The model under review builds one solid part; all positions refer to its coordinate system, in mm. A direction names the side the tool comes from. Coordinates: 2 decimals unless noted, no trailing zeros. Write each loop counter-clockwise with the first axis right and the second up, starting at its lowest first coordinate (ties: lowest second). Pieces come first, ordered by that corner, then holes. Notation, with made-up numbers: (60.5, 65.5) -> (66.5, 65.5) arc R32 cw to (66.5, 98.5) -> close; hole circle Ø2 at (46, -18.75). An arc over 180 degrees is marked (long way). Put each result on its own line as item: value. Start each with the question number.
Autodesk Inventor part; units mm, degrees
ref_plane "YZ Plane" through (0, 0, 0) normal (1, 0, 0) x (0, 1, 0)
ref_plane "XZ Plane" through (0, 0, 0) normal (0, 1, 0) x (-1, 0, 0)
ref_plane "XY Plane" through (0, 0, 0) normal (0, 0, 1) x (1, 0, 0)
sketch "Sketch1" plane through (0, 0, 0) normal (0, 0, 1) x (1, 0, 0)
  line L0 (0, 0) -> (-22, 0)
  line L1 (-22, 0) -> (-22, -15.6)
  line L2 (-22, -15.6) -> (-19, -15.6)
  line L3 (-19, -15.6) -> (-19, -5)
  line L4 (-19, -5) -> (-10, -5)
  line L5 (-10, -5) -> (-10, -2)
  line L6 (-10, -2) -> (0, -2)
  line L7 (0, -2) -> (0, 0)
  dimension "d0" = 2
  dimension "d1" = 10
  dimension "d2" = 3
  dimension "d3" = 9
  dimension "d4" = 3
  dimension "d5" = 10.6
extrude "Extrusion1" add sketch "Sketch1" along normal blind 10
chamfer "Chamfer1" distance 2 angle 45 1 edges at (-19, -5, 5)
sketch "Sketch2" plane through (-22, 0, 0) normal (0, 1, 0) x (1, 0, 0)
  line L0 (12, 0) -> (12, -10)
  line L1 (16.25, -5) -> (17.75, -5) construction
  line L2 (16.25, -6.75) -> (17.75, -6.75)
  line L3 (17.75, -3.25) -> (16.25, -3.25)
  arc A0 (16.25, -3.25) -> (16.25, -6.75) centre (16.25, -5) ccw
  arc A1 (17.75, -6.75) -> (17.75, -3.25) centre (17.75, -5) ccw
  point P0 (22, 0)
  point P1 (17, -5)
  dimension "d11" = 1.75
  dimension "d12" = 1.5
  dimension "d13" = 5
extrude "Extrusion2" cut sketch "Sketch2" against normal through all
chamfer "Chamfer2" distance 2 angle 45 1 edges at (-22, 0, 5)
chamfer "Chamfer3" distance 1 angle 45 8 edges at (-10, 0, 10) (-10, 0, 0) (0, 0, 5) (-21, -1, 10) (-22, -8.8, 10) (-21, -1, 0) (-22, -8.8, 0) (-22, -15.6, 5)
properties part number "_3DPrint"
1. Consider section A-A on z = 5. State the section outline as (x, y) points, then the cut area to 3 significant figures.
2. Consider section D-D on z = 2. State the section outline as (x, y) points, then the cut area to 3 significant figures.
3. Consider section C-C on x = -1.75. State the section outline as (y, z) points, then the cut area to 3 significant figures.
4. Insertion check: P1, Ø4, axis at y = -12, z = 8.5, coming from the +X side; P2, Ø0.9, axis at y = -4, z = 6.5, coming from the +X side. Each pin has a flat end and moves straight along its axis. Give the tip position at first contact, or say it passes through.
5. Tool access review of faces 5 (the cylindrical face through (-2.5, -1, 5)), 6 (the flat face through (-0.5, -0.5, 4.9)), 7 (the flat face through (-19, -11, 5)): name each direction out of +Z, -Z, +X, -X, +Y, -Y from which nothing blocks a thin tool from reaching the whole face with its end or side.
6. Wall thickness on line 1 (X direction, y = -4, z = 7); line 2 (X direction, y = -13, z = 4); line 3 (Y direction, x = -15.5, z = 2.25): over which ranges is each line inside the solid? List them lowest first. Write a range as from..to.
7. The part is to be moulded in two halves that separate along Z. For faces 1 (the flat face through (-16, -4, 0)), 2 (the flat face through (-22, -8, 5)), 3 (the flat face through (-21.5, -8.9, 9.5)), 4 (the cylindrical face through (-7.5, -1, 5)), say which applies: released by +Z, released by -Z, zero draft, split by the parting line, or undercut.
8. Consider section B-B on y = -8. State the section outline as (x, z) points.
Output values:
1. outline: (-22, -14.6) -> (-21, -15.6) -> (-19, -15.6) -> (-19, -7) -> (-17, -5) -> (-10, -5) -> (-10, -2) -> (-7.5, -2) -> (-7.5, 0) -> (-20, 0) -> (-22, -2) -> close; (-2.5, -2) -> (0, -2) -> (0, -1) -> (-1, 0) -> (-2.5, 0) -> close
1. area: 101 mm^2
2. outline: (-22, -14.6) -> (-21, -15.6) -> (-19, -15.6) -> (-19, -7) -> (-17, -5) -> (-10, -5) -> (-10, -2) -> (0, -2) -> (0, -1) -> (-1, 0) -> (-20, 0) -> (-22, -2) -> close
2. area: 111 mm^2
3. outline: (-2, 0) -> (-1, 0) -> (0, 1) -> (0, 9) -> (-1, 10) -> (-2, 10) -> close
3. area: 19.0 mm^2
4. P1: stops at x = -19
4. P2: stops at x = -10
5. face 5: +Y, -Y
5. face 6: +Z, -Z, +X, +Y
5. face 7: +Z, -Z, +X, -Y
6. line 1: x = -22..-10
6. line 2: x = -22..-19
6. line 3: y = -5..0
7. face 1: released by -Z
7. face 2: zero draft
7. face 3: released by +Z
7. face 4: undercut
8. outline: (-22, 1) -> (-21, 0) -> (-19, 0) -> (-19, 10) -> (-21, 10) -> (-22, 9) -> close
